Geometry check sheet. Reference: the model listing, model coordinates, mm. A direction names the side the tool comes from. Give positions to 0.01 mm unless a question says otherwise; leave off trailing zeros. Loops run counter-clockwise (first coordinate to the right, second up) from the corner with the lowest first, then second, coordinate; pieces in that order, holes last. Notation, with made-up numbers: (18.5, -10.5) -> (42.5, -10.5) arc R36 ccw to (42.5, 27.5) -> close; hole circle Ø6 at (55, -36.75). An arc over 180 degrees is marked (long way). Answer in a Markdown table with one row per item. Add a question column.
```python
from build123d import *

# Parameters (mm, degrees)
ESQUISSE1_W              = 305
ESQUISSE1_H              = 305
BOSS_EXTRU_1_DEPTH       = 180
ESQUISSE2_R              = 10
ENL_V_MAT_EXTRU_10_DEPTH = 10
CONG_2_R                 = 15
ENL_V_MAT_EXTRU_11_DEPTH = 180


with BuildPart() as part:
    # Esquisse1 → Boss.-Extru.1 (new body)
    with BuildSketch(Plane.XY):
        Rectangle(ESQUISSE1_W, ESQUISSE1_H)
    extrude(amount=BOSS_EXTRU_1_DEPTH)

    # Esquisse2 → Enlèv. mat.-Extru.10 (cut)
    with BuildSketch(Plane.XY.offset(180)):
        with Locations((137.5, 137.5)):
            Circle(ESQUISSE2_R)
        with Locations((137.5, -137.5)):
            Circle(ESQUISSE2_R)
        with Locations((-137.5, -137.5)):
            Circle(ESQUISSE2_R)
        with Locations((-137.5, 137.5)):
            Circle(ESQUISSE2_R)
    extrude(amount=-ENL_V_MAT_EXTRU_10_DEPTH, mode=Mode.SUBTRACT)

    # Congé2
    cong_2_edges = [part.edges().sort_by_distance(p)[0] for p in [
        (-152.5, 152.5, 90),
        (152.5, 152.5, 90),
        (152.5, -152.5, 90),
        (-152.5, -152.5, 90),
    ]]
    fillet(cong_2_edges, radius=CONG_2_R)

    # Esquisse3 → Enlèv. mat.-Extru.11 (cut)
    with BuildSketch(Plane.XY.offset(180)):
        with BuildLine():
            Line((-137.5, 147.5), (137.5, 147.5))
            ThreePointArc((137.5, 147.5), (144.571068, 144.571068), (147.5, 137.5))
            Line((147.5, 137.5), (147.5, -137.5))
            ThreePointArc((147.5, -137.5), (144.571068, -144.571068), (137.5, -147.5))
            Line((137.5, -147.5), (-137.5, -147.5))
            ThreePointArc((-137.5, -147.5), (-144.571068, -144.571068), (-147.5, -137.5))
            Line((-147.5, -137.5), (-147.5, 137.5))
            ThreePointArc((-147.5, 137.5), (-144.571068, 144.571068), (-137.5, 147.5))
        make_face()
    extrude(amount=-ENL_V_MAT_EXTRU_11_DEPTH, mode=Mode.SUBTRACT)


solid = part.part
```
1. Access from +Z, -Z, +X, -X, +Y, -Y to the whole of each face (thin tool, end or side, straight path). Record for faces 4 (the face through (-2, -152.5, 89)), 5 (the face through (-2, 147.5, 91)).
2. Release check for a two-part mould opening along Y. For faces 1 (the face through (-68, 148, 0)), 2 (the face through (-2, 152.5, 89)), 3 (the face through (2, -147.5, 91)) record: released by +Y, released by -Y, zero draft, split by the parting line, or undercut.
3. Sectioned sample at A-A (y = 101). Enter the section's corners in (x, z), plus the area to 3 significant figures.
4. Material ranges on L1, parallel to Y at x = -23, z = 129, recorded low to high. Write a range as from..to.
5. Sectioned sample at B-B (z = 111). Enter the section's corners in (x, y).
Response:
| question | item | result |
|---|---|---|
| 1 | face 4 | +Z, -Z, +X, -X, -Y |
| 1 | face 5 | +Z, -Z |
| 2 | face 1 | zero draft |
| 2 | face 2 | released by +Y |
| 2 | face 3 | undercut |
| 3 | outline | (-152.5, 0) -> (-147.5, 0) -> (-147.5, 180) -> (-152.5, 180) -> close; (147.5, 0) -> (152.5, 0) -> (152.5, 180) -> (147.5, 180) -> close |
| 3 | area | 1,800 mm2 |
| 4 | L1 | y = -152.5..-147.5, 147.5..152.5 |
| 5 | outline | (-152.5, -137.5) arc R15 ccw to (-137.5, -152.5) -> (137.5, -152.5) arc R15 ccw to (152.5, -137.5) -> (152.5, 137.5) arc R15 ccw to (137.5, 152.5) -> (-137.5, 152.5) arc R15 ccw to (-152.5, 137.5) -> close; hole (-147.5, -137.5) arc R10 ccw to (-137.5, -147.5) -> (137.5, -147.5) arc R10 ccw to (147.5, -137.5) -> (147.5, 137.5) arc R10 ccw to (137.5, 147.5) -> (-137.5, 147.5) arc R10 ccw to (-147.5, 137.5) -> close |
